```python
from build123d import *

# Parameters (mm, degrees)
SKETCH_1_R          = 10
EXTRUDE_1_DEPTH     = 5
SKETCH_2_R          = 6
EXTRUDE_2_DEPTH     = 4
SKETCH_3_W          = 12.239393476
SKETCH_3_H          = 3.581573668
CUT_EXTRUDE_1_DEPTH = 0.2


with BuildPart() as part:
    # 草图1 → 凸台-拉伸1 (new body)
    with BuildSketch(Plane(origin=(0, 0, 0), x_dir=(1, 0, 0), z_dir=(0, 1, 0))):
        with Locations(Location((0, 0, 0), (0, 0, 270))):
            Circle(SKETCH_1_R)
    extrude(amount=EXTRUDE_1_DEPTH)

    # 草图2 → 凸台-拉伸2 (add)
    with BuildSketch(Plane.XZ):
        with Locations(Location((0, 0, 0), (0, 0, 270))):
            Circle(SKETCH_2_R)
    extrude(amount=EXTRUDE_2_DEPTH)

    # 草图3 → 切除-拉伸1 (cut)
    with BuildSketch(Plane(origin=(0, 5, 0), x_dir=(1, 0, 0), z_dir=(0, 1, 0))):
        Rectangle(SKETCH_3_W, SKETCH_3_H)
    extrude(amount=-CUT_EXTRUDE_1_DEPTH, mode=Mode.SUBTRACT)


solid = part.part
```
Input: part model. Units: mm. Frame: model coordinates. A direction names the side the tool comes from. Give positions to 0.01 mm unless a question says otherwise; leave off trailing zeros. Loops run counter-clockwise (first coordinate to the right, second up) from the corner with the lowest first, then second, coordinate; pieces in that order, holes last. Notation, with made-up numbers: M -37.5,12 L 19.5,12 A15 cw 19.5,17 Z; hole C 58.5,66.5 d6. An arc over 180 degrees is marked long. Answer as CSV lines item,"result". Start each with the question number.
1. Section A-A on x = 0. Return loops of the section in (y, z), plus the area to 3 significant figures.
2. Section C-C on y = 2.5. Return loops of the section in (x, z).
3. Reachability of faces 1 (the face through (1.802, -1.972, -5.723)), 2 (the face through (0, -4, 0)) from +Z, -Z, +X, -X, +Y, -Y: full face, straight path, thin tool, end or side. Return the list, or none.
4. Section B-B on z = -2.5. Return loops of the section in (x, y).
5. Pull-direction query (Z, two-part tool) for faces 3 (the face through (0, 4.8, 0)), 4 (the face through (-9.76, 2.46, -2.17)), 5 (the face through (0, 5, 2)); classes: released by +Z, released by -Z, zero draft, split by the parting line, or undercut.
6. Pin query (flat end, axial travel): P1, Ø4, axis at x = -3, z = 0, coming from the +Y side; P2, Ø5, axis at y = -1.5, z = -4.5, coming from the -X side; P3, Ø3, axis at x = 2.5, y = 1.5, coming from the +Z side; P4, Ø2, axis at y = 3.5, z = -7.5, coming from the -X side. Return the tip coordinate at first contact, or that it passes through.
7. Section D-D on z = 0. Return loops of the section in (x, y), plus the area to 3 significant figures.
8. Line query: L1, parallel to Y at x = -6, z = -1.5; L2, parallel to Y at x = 7.75, z = 5; L3, parallel to X at y = -3.5, z = 3.5. Output: solid intervals per line, ascending.
Computed values:
1,outline,"M -4,-6 L 0,-6 L 0,-10 L 5,-10 L 5,-1.79 L 4.8,-1.79 L 4.8,1.79 L 5,1.79 L 5,10 L 0,10 L 0,6 L -4,6 Z"
1,area,"147 mm²"
2,outline,"C 0,0 d20"
3,face 1,"-Y"
3,face 2,"+Z, -Z, +X, -X, -Y"
4,outline,"M -9.68,0 L -5.45,0 L -5.45,-4 L 5.45,-4 L 5.45,0 L 9.68,0 L 9.68,5 L -9.68,5 Z"
5,face 3,"undercut"
5,face 4,"split by the parting line"
5,face 5,"zero draft"
6,P1,"stops at y = 5"
6,P2,"stops at x = -9.68"
6,P3,"stops at z = 9.95"
6,P4,"stops at x = -7.6"
7,outline,"M -10,0 L -6,0 L -6,-4 L 6,-4 L 6,0 L 10,0 L 10,5 L 6.12,5 L 6.12,4.8 L -6.12,4.8 L -6.12,5 L -10,5 Z"
7,area,"146 mm²"
8,L1,"y = 0 to 4.8"
8,L2,"y = 0 to 5"
8,L3,"x = -4.87 to 4.87"
